Input: part model. Units: mm. Frame: model coordinates. A direction names the side the tool comes from. Coordinates: 2 decimals unless noted, no trailing zeros. Write each loop counter-clockwise with the first axis right and the second up, starting at its lowest first coordinate (ties: lowest second). Pieces come first, ordered by that corner, then holes. Notation, with made-up numbers: (13, 63) - (55, 63) arc R21 cw to (55, 78) - close; hole circle Ø6 at (43, 62). An arc over 180 degrees is marked (long way). Use a Markdown table: item, result. Add a question column.
Q1. Section query C-C (y = -95.5). Return the cut outline in (x, z), then the cut area to 3 significant figures.
Q2. Pin query (flat end, axial travel): P1, Ø3, axis at y = -63, z = -15, coming from the -X side; P2, Ø1, axis at x = -86, z = -24.5, coming from the +Y side; P3, Ø10, axis at x = 7.5, z = -19.5, coming from the +Y side. Return the tip coordinate at first contact, or that it passes through.
Q3. Mould query, pull axis X, two halves, no side actions, for faces 4 (the face through (-59.6, -3, 1.5)), 5 (the face through (-54.657, 134.148, 1.479)), 6 (the face through (-2, 33, 3)). Classes: released by +X, released by -X, zero draft, split by the parting line, or undercut.
Q4. Section query A-A (x = -97). Return the cut outline in (y, z).
Q5. Material intervals for probe 1 along Z at (x, y) = (65.5, -99); probe 2 along X at (y, z) = (-51.5, -5.5); probe 3 along Y at (x, z) = (-47.5, -12.5), sorted ascending. Write a range as from..to.
Q6. Section query D-D (y = -49.5). Return the cut outline in (x, z).
Q7. Set-up query: faces 1 (the face through (32.23, 13.65, 1.48)), 2 (the face through (133.505, -56.209, 1.479)), 3 (the face through (-40.77, -41.82, -17.74)). Return all of +Z, -Z, +X, -X, +Y, -Y with unobstructed straight access to the full face (end or side cutting, diameter ignored); none if empty.
Q8. Section query B-B (z = -24). Return the cut outline in (x, y), then the cut area to 3 significant figures.
from build123d import *

# Parameters (mm, degrees)
BOSS_EXTRUDE4_DEPTH = 3
BOSS_EXTRUDE5_START = -179.852814
SKETCH7_W           = 3
SKETCH7_H           = 35
BOSS_EXTRUDE5_DEPTH = 179.852814


with BuildPart() as part:
    # Sketch6 → Boss-Extrude4 (new body)
    with BuildSketch(Plane(origin=(0, 0, 0), x_dir=(0, 1, 0), z_dir=(0, 0, 1))):
        Polygon((156.787555785, 0), (110.865543901, 110.865543901), (0, 156.787555785), (-36.922845517, 141.493612411), (31.903846567, -24.66872107), (-5.116006301, -40.002846205), (-73.942698385, 126.159487276), (-110.865543901, 110.865543901), (-156.787555785, 0), (-110.865543901, -110.865543901), (0, -156.787555785), (110.865543901, -110.865543901), align=None)
    extrude(amount=BOSS_EXTRUDE4_DEPTH)

    # Sketch7 → Boss-Extrude5 (add)
    with BuildSketch(Plane(origin=(-133.826549843, -55.432771951, 0), x_dir=(0.38268343236508956, -0.9238795325112868, 0), z_dir=(-0.9238795325112868, -0.38268343236508956, 0)).offset(BOSS_EXTRUDE5_START)):
        with Locations((21.535, -17.5)):
            Rectangle(SKETCH7_W, SKETCH7_H)
    extrude(amount=BOSS_EXTRUDE5_DEPTH)


solid = part.part
Values follow:
| question | item | result |
|---|---|---|
| 1 | outline | (-117.23, 0) - (117.23, 0) - (117.23, 3) - (-117.23, 3) - close |
| 1 | area | 703 mm2 |
| 2 | P1 | x = -103.36 |
| 2 | P2 | y = -57.1 |
| 2 | P3 | y = -16.51 |
| 3 | face 4 | undercut |
| 3 | face 5 | released by -X |
| 3 | face 6 | zero draft |
| 4 | outline | (-116.61, 0) - (-65.11, 0) - (-65.11, -35) - (-61.86, -35) - (-61.86, 3) - (-116.61, 3) - close; (-18.49, 0) - (116.61, 0) - (116.61, 3) - (-18.49, 3) - close |
| 5 | probe 1 | 0..3 |
| 5 | probe 2 | -71.98..-64.14 |
| 5 | probe 3 | -44.61..-41.36 |
| 6 | outline | (-67.15, -35) - (-59.31, -35) - (-59.31, 0) - (136.28, 0) - (136.28, 3) - (-67.15, 3) - close |
| 7 | face 1 | +Z, -Z |
| 7 | face 2 | +Z, -Z, +X, -Y |
| 7 | face 3 | -Z, +X, -Y |
| 8 | outline | (-126.16, -73.94) - (-125.01, -76.71) - (41.15, -7.89) - (40, -5.12) - close |
| 8 | area | 540 mm2 |
